CAD build for the part. Positions are in the model's coordinates, mm. A direction names the side the tool comes from. Give positions to 0.01 mm unless a question says otherwise; leave off trailing zeros. Write each loop counter-clockwise with the first axis right and the second up, starting at its lowest first coordinate (ties: lowest second). Pieces come first, ordered by that corner, then holes. Notation, with made-up numbers: (27.5, -4.5) - (49.5, -4.5) arc R18 ccw to (49.5, 30.5) - close; hole circle Ø5 at (82, 69.25). An arc over 180 degrees is marked (long way). Write item = value, one per line. Start each with the question number.
Autodesk Inventor part; units mm, degrees
ref_plane "YZ Plane" through (0, 0, 0) normal (1, 0, 0) x (0, 1, 0)
ref_plane "XZ Plane" through (0, 0, 0) normal (0, 1, 0) x (-1, 0, 0)
ref_plane "XY Plane" through (0, 0, 0) normal (0, 0, 1) x (1, 0, 0)
sketch "Sketch1" plane through (0, 0, 0) normal (0, 1, 0) x (-1, 0, 0)
  line L0 (50, 50) -> (0, 50)
  line L1 (0, 50) -> (0, 0)
  line L2 (0, 0) -> (50, 0)
  line L3 (50, 0) -> (50, 50)
  line L4 (45, 45) -> (5, 45)
  line L5 (5, 45) -> (5, 5)
  line L6 (5, 5) -> (45, 5)
  line L7 (45, 5) -> (45, 45)
  line L8 (45, 5) -> (50, 5)
  line L9 (5, 45) -> (5, 50)
  dimension "d0" = 50
  dimension "d1" = 50
  dimension "d2" = 5
extrude "Extrusion1" add sketch "Sketch1" along normal blind 340 contours L9 L5 L6 L8 L3 L2 L1 L0
properties part number "Ugolok"
1. Cut at C-C (z = 31). Give the cut face in (x, y), then the cut area to 3 significant figures.
2. Pin check, flat tips, straight feed: pin 1 Ø10 at (y, z) = (266, 41.5) entering from -X; pin 2 Ø1.5 at (x, y) = (-18, 104) entering from +Z; pin 3 Ø1 at (x, y) = (-30, 182.5) entering from -Z. Stop position of each tip, or through.
3. Wall check: line 1 along X through (y, z) = (298, 7.5); line 2 along Z through (x, y) = (-36, 207.5). Give the ranges that are in metal, low to high.
4. Cut at B-B (x = -30). Give the cut face in (y, z).
5. Cut at A-A (y = 85.5). Give the cut face in (x, z), then the cut area to 3 significant figures.
6. Tool access for faces 1 (the flat face through (-27, 168, 5)), 2 (the flat face through (-13.8, 0, 4.7)): list every direction of +Z, -Z, +X, -X, +Y, -Y with a clear straight run to the whole face (end or side of a thin tool).
Output:
q1.outline = (-5, 0) - (0, 0) - (0, 340) - (-5, 340) - close
q1.area = 1,700 mm2
q2.pin_1 = -5
q2.pin_2 = 5
q2.pin_3 = 0
q3.line_1 = -5 to 0
q3.line_2 = 0 to 5
q4.outline = (0, 0) - (340, 0) - (340, 5) - (0, 5) - close
q5.outline = (-50, 0) - (0, 0) - (0, 50) - (-5, 50) - (-5, 5) - (-50, 5) - close
q5.area = 475 mm2
q6.face_1 = +Z, -X, +Y, -Y
q6.face_2 = +Z, -Z, +X, -X, -Y
